Could you check a few things on this model? Use its own coordinates, in mm. A direction names the side the tool comes from. Give positions to 0.01 mm unless a question says otherwise; leave off trailing zeros. Order: outer loops, then holes, each group sorted by start corner. A loop starts at its lowest first (then second) coordinate and runs counter-clockwise, first axis right, second up. Notation, with made-up numbers: (-25, 31.25) -> (-11, 31.25) arc R16 ccw to (-11, 51.25) -> close; hole circle Ø11 at (-22.75, 47). An arc over 180 degrees is marked (long way). One line per item, written item: value.
```python
from build123d import *

# Parameters (mm, degrees)
BOSS_EXTRUDE1_DEPTH = 76.2
SKETCH3_R           = 4.064
BOSS_EXTRUDE2_DEPTH = 6.35
SKETCH2_W           = 25.4
SKETCH2_H           = 6.35
CUT_EXTRUDE2_DEPTH  = 25.4


with BuildPart() as part:
    # Sketch1 → Boss-Extrude1 (new body)
    with BuildSketch(Plane(origin=(0, 0, 0), x_dir=(1, 0, 0), z_dir=(0, 1, 0))):
        Polygon((0, 0), (-25.4, 43.994090512), (25.4, 43.994090512), align=None)
    extrude(amount=BOSS_EXTRUDE1_DEPTH)

    # Sketch3 → Boss-Extrude2 (add)
    with BuildSketch(Plane(origin=(0, 76.2, 0), x_dir=(1, 0, 0), z_dir=(0, 1, 0))):
        with Locations((0, 29.329393675)):
            Circle(SKETCH3_R)
    extrude(amount=BOSS_EXTRUDE2_DEPTH)

    # Sketch2 → Cut-Extrude2 (cut)
    with BuildSketch(Plane(origin=(0, 0, 0), x_dir=(1, 0, 0), z_dir=(0, 1, 0))):
        with Locations((0, 29.329393675)):
            Rectangle(SKETCH2_W, SKETCH2_H)
    extrude(amount=CUT_EXTRUDE2_DEPTH, mode=Mode.SUBTRACT)


solid = part.part
```
1) Suppose I cut it at B-B, the plane z = -14. Write out the boundary of the cut face in (x, y).
Answer below:
outline: (-8.08, 0) -> (8.08, 0) -> (8.08, 76.2) -> (-8.08, 76.2) -> close
2) Suppose I cut it at C-C, the plane y = 62. Write out the boundary of the cut face in (x, z).
Answer below:
outline: (-25.4, -43.99) -> (25.4, -43.99) -> (0, 0) -> close
3) If I drill on line 1 along Y through (x, z) = (16.5, -30); line 2 along Z through (x, y) = (-5, 21.5); line 3 along Z through (x, y) = (-2, 20), over which ranges is the centre line in solid material (lowest first)?
Answer below:
line 1: y = 0 to 76.2
line 2: z = -43.99 to -32.5, -26.15 to -8.66
line 3: z = -43.99 to -32.5, -26.15 to -3.46
4) Suppose I cut it at D-D, the plane z = -34.5. Write out the boundary of the cut face in (x, y), then the cut area to 3 significant figures.
Answer below:
outline: (-19.92, 0) -> (19.92, 0) -> (19.92, 76.2) -> (-19.92, 76.2) -> close
area: 3,040 mm2
5) Suppose I cut it at A-A, the plane y = 15.5. Write out the boundary of the cut face in (x, z), then the cut area to 3 significant figures.
Answer below:
outline: (-25.4, -43.99) -> (25.4, -43.99) -> (0, 0) -> close; hole (-12.7, -32.5) -> (12.7, -32.5) -> (12.7, -26.15) -> (-12.7, -26.15) -> close
area: 956 mm2
6) We'd pull the mould along X, two halves only. Please class faces 1 (the flat face through (12.88, 37.57, -22.31)), 2 (the flat face through (0, 25.4, -29)), 3 (the flat face through (0, 38, -43.994)): +X half, -X half, draft (parallel to the pull), parting line (faces both ways), or undercut.
Answer below:
face 1: +X half
face 2: undercut
face 3: draft
7) For faces 4 (the flat face through (0, 13, -26.154)), 5 (the cylindrical face through (2.18, 79.33, -32.76)), 6 (the flat face through (0, 0, -22)), which set-ups out of +Z, -Z, +X, -X, +Y, -Y let a thin tool reach every point of the face, with its end or its side?
Answer below:
face 4: -Y
face 5: +Y
face 6: +Z, -Z, +X, -X, -Y
8) For P1, Ø10, axis at y = 12.5, z = -12, coming from the -X side; P2, Ø1, axis at x = 0, y = 12, coming from the +Z side; P3, Ø7, axis at y = 15, z = -29.5, coming from the +X side, each with a flat end and sliding along its axis, tell me the tip position at first contact or that it passes through.
Answer below:
P1: stops at x = -9.81
P2: stops at z = 0
P3: stops at x = 19.05
